```python
from build123d import *

# Parameters (mm, degrees)
SKETCH_1_W          = 15.4
SKETCH_1_H          = 22.4
EXTRUDE_2_DEPTH     = 3
EXTRUDE_3_DEPTH     = 5
EXTRUDE_3_2_DEPTH   = 5
EXTRUDE_4_DEPTH     = 15
SKETCH_3_R          = 1.55
CUT_EXTRUDE_2_DEPTH = 31.8
SKETCH_9_R          = 1.6
CUT_EXTRUDE_6_DEPTH = 16
SKETCH_10_R         = 3
CUT_EXTRUDE_7_DEPTH = 2
SKETCH_11_R         = 3
CUT_EXTRUDE_8_DEPTH = 2
CUT_EXTRUDE_9_DEPTH = 23.4


with BuildPart() as part:
    # Sketch 1 → Extrude 2 (new body)
    with BuildSketch(Plane(origin=(0, 0, 0), x_dir=(1, 0, 0), z_dir=(0, 1, 0))):
        Rectangle(SKETCH_1_W, SKETCH_1_H)
    extrude(amount=EXTRUDE_2_DEPTH)



with BuildPart() as body_2:
    # Sketch 1_4 → Extrude 3 (new body)
    with BuildSketch(Plane(origin=(0, 0, 0), x_dir=(1, 0, 0), z_dir=(0, 1, 0))):
        Polygon((7.7, -11.2), (7.7, -7.7), (0, -7.7), (-4.7, -7.7), (-7.7, -7.7), (-7.7, -11.2), align=None)
    extrude(amount=EXTRUDE_3_DEPTH)


with BuildPart() as body_3:
    # Sketch 1_4 → Extrude 3 2 (new body)
    with BuildSketch(Plane(origin=(0, 0, 0), x_dir=(1, 0, 0), z_dir=(0, 1, 0))):
        Polygon((-7.7, 7.7), (0, 7.7), (7.7, 7.7), (7.7, 11.2), (-7.7, 11.2), align=None)
    extrude(amount=EXTRUDE_3_2_DEPTH)


with BuildPart() as part_1:
    add(part.part)

    add(body_2.part)  # Extrude 4 merges body 2

    add(body_3.part)  # Extrude 4 merges body 3
    # Sketch 1_5 → Extrude 4 (add)
    with BuildSketch(Plane(origin=(0, 0, 0), x_dir=(1, 0, 0), z_dir=(0, 1, 0))):
        Polygon((-7.7, 0), (-7.7, 7.7), (-7.7, 11.2), (-11.2, 11.2), (-11.2, -11.2), (-7.7, -11.2), (-7.7, -7.7), align=None)
        Polygon((7.7, 11.2), (7.7, 7.7), (7.7, 0), (7.7, -7.7), (7.7, -11.2), (11.2, -11.2), (11.2, 11.2), align=None)
        Polygon((7.7, -11.2), (7.7, -7.7), (0, -7.7), (-4.7, -7.7), (-7.7, -7.7), (-7.7, -11.2), align=None)
        Polygon((-7.7, 7.7), (0, 7.7), (7.7, 7.7), (7.7, 11.2), (-7.7, 11.2), align=None)
    extrude(amount=EXTRUDE_4_DEPTH)

    # Sketch 3 → Cut-Extrude 2 (cut, through all)
    with BuildSketch(Plane(origin=(0, 0, -19.6), x_dir=(-1, 0, 0), z_dir=(0, 0, -1))):
        with Locations((0, 10)):
            Circle(SKETCH_3_R)
    extrude(amount=-CUT_EXTRUDE_2_DEPTH, mode=Mode.SUBTRACT)

    # Sketch 9 → Cut-Extrude 6 (cut, through all)
    with BuildSketch(Plane.XZ):
        with Locations((0, 4)):
            Circle(SKETCH_9_R)
        with Locations((0, -4)):
            Circle(SKETCH_9_R)
    extrude(amount=-CUT_EXTRUDE_6_DEPTH, mode=Mode.SUBTRACT)

    # Sketch 10 → Cut-Extrude 7 (cut)
    with BuildSketch(Plane(origin=(0, 0, -11.2), x_dir=(-1, 0, 0), z_dir=(0, 0, -1))):
        with Locations((0, 10)):
            Circle(SKETCH_10_R)
    extrude(amount=-CUT_EXTRUDE_7_DEPTH, mode=Mode.SUBTRACT)

    # Sketch 11 → Cut-Extrude 8 (cut)
    with BuildSketch(Plane.XY.offset(11.2)):
        with Locations((0, 10)):
            Circle(SKETCH_11_R)
    extrude(amount=-CUT_EXTRUDE_8_DEPTH, mode=Mode.SUBTRACT)

    # Sketch 8 → Cut-Extrude 9 (cut, through all)
    with BuildSketch(Plane.ZY.offset(11.2)):
        Polygon((7.5, 10), (7.5, 3), (0, 3), (-7.5, 3), (-7.5, 13), (7.5, 13), align=None)
    extrude(amount=-CUT_EXTRUDE_9_DEPTH, mode=Mode.SUBTRACT)


solid = part_1.part
```
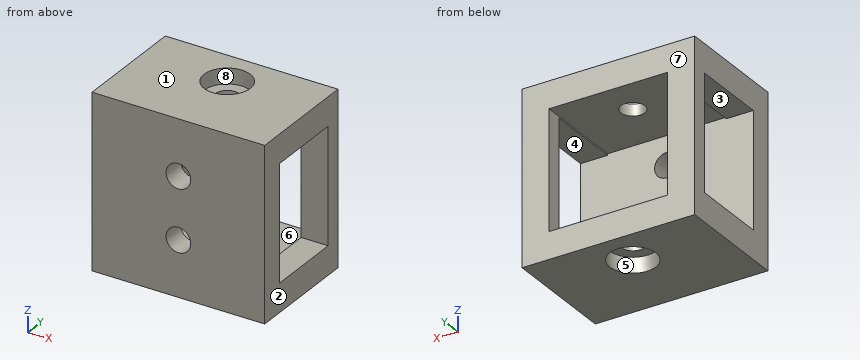
Input: part model. Units: mm. Frame: model coordinates. Face numbers are marked on the shaded views. A direction names the side the tool comes from. Coordinates: 2 decimals unless noted, no trailing zeros. Loops run counter-clockwise (first coordinate to the right, second up) from the corner with the lowest first, then second, coordinate; pieces in that order, holes last. Notation, with made-up numbers: M -34.5,20.5 L -25.5,20.5 A21 cw -25.5,43.5 Z; hole C 74.25,-16 d4. An arc over 180 degrees is marked long. Use a Markdown table: item, result. Add a question column.
1) Section B-B, the plane x = 0. Give the number of separate pieces and of enclosed holes in the cut face, plus the area to 3 significant figures.
2) Pin query (flat end, axial travel): P1, Ø4.5, axis at x = 4.5, z = 3, coming from the +Y side; P2, Ø1.8, axis at x = 0.5, y = 10.5, coming from the -Z side; P3, Ø3, axis at x = 0, y = 10, coming from the +Z side. Return the tip coordinate at first contact, or that it passes through.
3) Set-up query: the marked faces 4, 5, 6, 7 and 8. Return all of +Z, -Z, +X, -X, +Y, -Y with unobstructed straight access to the full face (end or side cutting, diameter ignored); none if empty.
4) Line query: L1, parallel to Z at x = -3, y = 11.5; L2, parallel to Z at x = 7.75, y = 9.5; L3, parallel to Y at x = 7.75, z = 7. Output: solid intervals per line, ascending. Write a range as from..to.
5) Section D-D, the plane y = 5.5. Return the cut outline in (x, z), plus the area to 3 significant figures.
6) Draft query along Z for the marked faces 1, 2 and 3. Return one class per face: +Z half, -Z half, draft (parallel to the pull), parting line (faces both ways), or undercut.
7) Section A-A, the plane z = 4. Return the cut outline in (x, y).
Answer below:
| question | item | result |
|---|---|---|
| 1 | separate pieces | 5 |
| 1 | enclosed holes | 0 |
| 1 | area | 98.7 mm2 |
| 2 | P1 | y = 3 |
| 2 | P2 | z = -9.2 |
| 2 | P3 | through |
| 3 | face 4 | +X, -X |
| 3 | face 5 | -Z |
| 3 | face 6 | +Y |
| 3 | face 7 | +Z, -Z, +X, -X, +Y |
| 3 | face 8 | +Z |
| 4 | L1 | -11.2..-7.7, 7.7..11.2 |
| 4 | L2 | -11.2..-7.5, 7.5..11.2 |
| 4 | L3 | 0..3, 13..15 |
| 5 | outline | M -11.2,-11.2 L 11.2,-11.2 L 11.2,-7.5 L 7.7,-7.5 L 7.7,-7.7 L -7.7,-7.7 L -7.7,-7.5 L -11.2,-7.5 Z; M -11.2,7.5 L -7.7,7.5 L -7.7,7.7 L 7.7,7.7 L 7.7,7.5 L 11.2,7.5 L 11.2,11.2 L -11.2,11.2 Z |
| 5 | area | 160 mm2 |
| 6 | face 1 | +Z half |
| 6 | face 2 | draft |
| 6 | face 3 | undercut |
| 7 | outline | M -11.2,0 L -1.6,0 L -1.6,3 L -11.2,3 Z; M -11.2,13 L -7.7,13 L -7.7,15 L -11.2,15 Z; M 1.6,0 L 11.2,0 L 11.2,3 L 1.6,3 Z; M 7.7,13 L 11.2,13 L 11.2,15 L 7.7,15 Z |
